Could you check a few things on this model? Use its own coordinates, in mm. Face numbers are marked on the shaded views. A direction names the side the tool comes from. Give positions to 0.01 mm unless a question says otherwise; leave off trailing zeros. Order: outer loops, then holes, each group sorted by start corner. A loop starts at its lowest first (then second) coordinate and runs counter-clockwise, first axis right, second up. Notation, with made-up numbers: (59.5, 24) - (109.5, 24) arc R12 ccw to (109.5, 47) - close; hole circle Ø3 at (-21.75, 30). An arc over 180 degrees is marked (long way). One line per question, with ' | ' between items. Start each with the question number.
1. Imagine slicing it at A-A (y = 0). Please give me the cut outline in (x, z), and give its area (3 significant figures).
2. I need wall thicknesses on probe 1 along Z at (x, y) = (-34, 0.5); probe 2 along X at (y, z) = (5.5, 0.5); probe 3 along X at (y, z) = (-6.25, 4.5). Which ranges of each line are inside material? Lowest first, please. Write a range as from..to.
3. For P1, Ø4, axis at x = -41, y = 4, coming from the +Z side; P2, Ø8, axis at x = 43, z = -5, coming from the +Y side; P3, Ø2, axis at x = -58, z = -5, coming from the +Y side, each with a flat end and sliding along its axis, tell me the tip position at first contact or that it passes through.
4. Which directions (+Z, -Z, +X, -X, +Y, -Y) give clear straight access to the entire face, cutting with the end or side of a thin tool? Please do the marked faces 1 and 2.
5. Imagine slicing it at C-C (x = 106.5). Please give me the cut outline in (y, z), and give its area (3 significant figures).
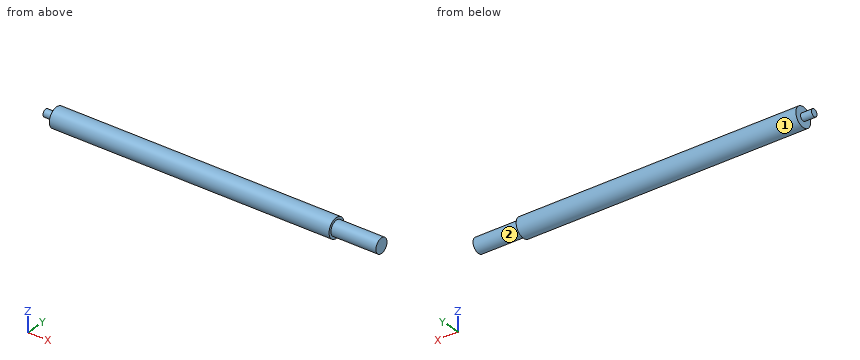
```python
from build123d import *

# Parameters (mm, degrees)
SKETCH_1_R      = 8
EXTRUDE_1_DEPTH = 115
SKETCH_2_R      = 6
EXTRUDE_2_DEPTH = 37
SKETCH_5_R      = 3
EXTRUDE_4_DEPTH = 9


with BuildPart() as part:
    # 草图1 → 凸台-拉伸1 (new, symmetric)
    with BuildSketch(Plane(origin=(0, 0, 0), x_dir=(0, 0, -1), z_dir=(1, 0, 0))):
        Circle(SKETCH_1_R)
    extrude(amount=EXTRUDE_1_DEPTH, both=True)

    # 草图2 → 凸台-拉伸2 (add)
    with BuildSketch(Plane(origin=(115, 0, 0), x_dir=(0, 0, -1), z_dir=(1, 0, 0))):
        Circle(SKETCH_2_R)
    extrude(amount=EXTRUDE_2_DEPTH)

    # 草图5 → 凸台-拉伸4 (add, symmetric)
    with BuildSketch(Plane.ZY.offset(115)):
        with Locations(Location((0, 0, 0), (0, 0, 180))):
            Circle(SKETCH_5_R)
    extrude(amount=EXTRUDE_4_DEPTH, both=True)


solid = part.part
```
Results found:
1) outline: (-124, -3) - (-115, -3) - (-115, -8) - (115, -8) - (115, -6) - (152, -6) - (152, 6) - (115, 6) - (115, 8) - (-115, 8) - (-115, 3) - (-124, 3) - close | area: 4,180 mm2
2) probe 1: z = -7.98..7.98 | probe 2: x = -115..152 | probe 3: x = -115..115
3) P1: stops at z = 7.75 | P2: stops at y = 7.94 | P3: stops at y = 6.93
4) face 1: +X, -X | face 2: +X
5) outline: circle Ø16 at (0, 0) | area: 201 mm2
